Autodesk Inventor part; units mm, degrees
ref_plane "YZ Plane" through (0, 0, 0) normal (1, 0, 0) x (0, 1, 0)
ref_plane "XZ Plane" through (0, 0, 0) normal (0, 1, 0) x (-1, 0, 0)
ref_plane "XY Plane" through (0, 0, 0) normal (0, 0, 1) x (1, 0, 0)
sketch "Sketch1" plane through (0, 0, 0) normal (0, 0, 1) x (1, 0, 0)
  line L0 (-131, -26) -> (-49, -26) construction
  line L1 (-49, -26) -> (-49, -52.5) construction
  line L2 (-49, -52.5) -> (-131, -52.5) construction
  line L3 (-131, -52.5) -> (-131, -26) construction
  line L4 (-90, -26) -> (-90, 12) construction
  line L5 (-140, -12) -> (-40, -12) construction
  line L6 (-40, -12) -> (-40, -62) construction
  line L7 (-40, -62) -> (-140, -62) construction
  line L8 (-140, -62) -> (-140, -12) construction
  line L9 (-140, -18) -> (-40, -18) construction
  line L10 (-90, -12) -> (-90, 12) construction
  line L11 (0, 0) -> (-90, 0) construction
  line L12 (-30, -17.3205) -> (0, 34.641)
  line L13 (0, 34.641) -> (30, -17.3205)
  line L14 (30, -17.3205) -> (-30, -17.3205)
  line L15 (0, -17.3205) -> (0, 34.641) construction
  line L16 (-15, 8.6603) -> (30, -17.3205) construction
  line L17 (15, 8.6603) -> (-30, -17.3205) construction
  line L18 (80.3923, -115.2436) -> (30.3923, -28.641) construction
  line L19 (123.6936, -90.2436) -> (80.3923, -115.2436) construction
  line L20 (73.6936, -3.641) -> (123.6936, -90.2436) construction
  line L21 (30.3923, -28.641) -> (73.6936, -3.641) construction
  line L22 (67.5167, -64.9423) -> (34.6077, -83.9423) construction
  line L23 (59.6077, 127.2436) -> (9.6077, 40.641) construction
  line L24 (16.3064, 152.2436) -> (59.6077, 127.2436) construction
  line L25 (-33.6936, 65.641) -> (16.3064, 152.2436) construction
  line L26 (9.6077, 40.641) -> (-33.6936, 65.641) construction
  line L27 (22.4833, 90.9423) -> (55.3923, 71.9423) construction
  line L28 (3.9859, 170.9038) -> (-45, 86.0577)
  line L29 (-45, 86.0577) -> (-45, -11)
  line L30 (-45, -11) -> (-150, -11)
  line L31 (-150, -11) -> (-150, -82)
  line L32 (-52.0282, -82) -> (32.0263, -33.4711)
  line L33 (84.5263, -124.4038) -> (146.0141, -88.9038)
  line L34 (32.0263, -33.4711) -> (84.5263, -124.4038)
  line L35 (-150, -82) -> (-52.0282, -82)
  line L36 (97.0282, -4.0577) -> (12.9737, 44.4711)
  line L37 (65.4737, 135.4038) -> (3.9859, 170.9038)
  line L38 (12.9737, 44.4711) -> (65.4737, 135.4038)
  line L39 (146.0141, -88.9038) -> (97.0282, -4.0577)
  point P0 (-90, -18)
  point P1 (55.3923, -71.9423)
  point P2 (85.5885, -112.2436)
  point P3 (35.5885, -25.641)
  point P4 (110.9663, -87.1993)
  point P5 (69.9663, -16.1852)
  point P6 (47.0167, -29.4352)
  point P7 (88.0167, -100.4493)
  point P8 (34.6077, 83.9423)
  point P9 (54.4115, 130.2436)
  point P10 (4.4115, 43.641)
  point P11 (20.0337, 139.6993)
  point P12 (-20.9663, 68.6852)
  point P13 (1.9833, 55.4352)
  point P14 (42.9833, 126.4493)
  point P15 (3.9859, 170.9038)
  point P16 (-150, -82)
  point P17 (146.0141, -88.9038)
  dimension "d0" = 26.5
  dimension "d1" = 82
  dimension "d2" = 9.5
  dimension "d3" = 100
  dimension "d4" = 50
  dimension "d5" = 6
  dimension "d6" = 30
  dimension "d7" = 90
  dimension "d8" = 60
  dimension "d11" = 360
  dimension "d13" = 20
  dimension "d14" = 1
  dimension "d15" = 10
  dimension "d16" = 20
  dimension "d17" = 10
  dimension "d18" = 5
  dimension "d21" = 360
extrude "Extrusion1" add sketch "Sketch1" along normal blind 6
hole "Hole1" at (-131, -26, 0) at (-49, -26, 0) at (-49, -52.5, 0) at (-131, -52.5, 0) at (110.9663, -87.1993, 0) at (69.9663, -16.1852, 0) at (47.0167, -29.4352, 0) at (88.0167, -100.4493, 0) at (20.0337, 139.6993, 0) at (-20.9663, 68.6852, 0) at (1.9833, 55.4352, 0) at (42.9833, 126.4493, 0) direction (0, 0, 1) diameter 6.6 end through all
chamfer "Chamfer1" distance 7.5 angle 45 3 edges at (32.0263, -33.4711, 3) (12.9737, 44.4711, 3) (-45, -11, 3)
fillet "Fillet1" radius 10 6 edges at (84.5263, -124.4038, 3) (146.0141, -88.9038, 3) (-52.0282, -82, 3) (35.7763, -39.9663, 3) (25.5311, -37.2211, 3) (30, -17.3205, 3)
pattern_circular "Circular Pattern1" count 3 over 360 about axis through (0, 0, -10) along (0, 0, 1) of "Fillet1"
sketch "Sketch2" plane through (0, 0, 6) normal (0, 0, 1) x (1, 0, 0)
  point P0 (0, 0)
sketch "Sketch3" plane through (0, 0, 0) normal (0, 0, -1) x (-1, 0, 0)
  line L0 (-94.7077, -2.718) -> (-23.0561, 38.6501)
  line L1 (-141.0141, -80.2436) -> (-98.3679, -6.3782)
  line L2 (-93.1865, -119.4038) -> (-137.3538, -93.9038)
  line L3 (-8.6603, 19.641) -> (-21.3397, -2.3205)
  line L4 (-37.8473, -43.5535) -> (-79.5263, -115.7436)
  line L5 (-18.7948, 54.5535) -> (-60.4737, 126.7436)
  line L6 (-123.6936, -90.2436) -> (-113.6936, -72.923)
  line L7 (-113.6936, -72.923) -> (-131.0141, -62.923)
  line L8 (-131.0141, -62.923) -> (-141.0141, -80.2436)
  line L9 (-141.0141, -80.2436) -> (-123.6936, -90.2436)
  line L10 (-123.6936, -90.2436) -> (-131.0141, -62.923) construction
  line L11 (-113.6936, -72.923) -> (-141.0141, -80.2436) construction
  point P0 (0, 0)
  point P1 (-117.3538, -59.2628)
  point P2 (-127.3538, -76.5833)
  point P3 (-33.9545, 20.8109)
  point P4 (-16.634, 30.8109)
  point P5 (-38.6603, -12.3205)
  dimension "d39" = 10
  dimension "d40" = 10
  dimension "d41" = 20
  dimension "d42" = 20
  dimension "d43" = 10
  dimension "d44" = 10
  dimension "d46" = 10
  dimension "d47" = 20
  dimension "d49" = 120
  dimension "d50" = 30
  dimension "d58" = 20
  dimension "d59" = 20
hole "Hole2" at (38.6603, -12.3205, 0) at (33.9545, 20.8109, 0) at (16.634, 30.8109, 0) at (127.3538, -76.5833, 0) at (117.3538, -59.2628, 0) direction (0, 0, 1) diameter 5.5 end through all
pattern_circular "Circular Pattern2" count 3 over 360 about axis through (0, 0, -10) along (0, 0, 1) of "Hole2"
properties part number "RT_FRM_MC_V3_MotorBase"
Model file for the job. Use its own axes, mm. A direction names the side the tool comes from. Give positions to 0.01 mm unless a question says otherwise; leave off trailing zeros. Loops run counter-clockwise (first coordinate to the right, second up) from the corner with the lowest first, then second, coordinate; pieces in that order, holes last. Notation, with made-up numbers: (-22.5, -24) - (36.5, -24) arc R29 cw to (36.5, 11) - close; hole circle Ø9 at (89.5, 62). An arc over 180 degrees is marked (long way). Use one line per item in the form item = value.
(1) Cut at C-C (x = -99.5). Give the cut face in (y, z), then the cut area to 3 significant figures.
Determined:
outline = (-82, 0) - (-11, 0) - (-11, 6) - (-82, 6) - close
area = 426 mm^2
(2) Pull direction X, two halves, no side cores. Call faces 5 (the face through (-127.78, -53.22, 3.04)), 6 (the face through (-147.15, -78.99, 3.04)), 7 (the face through (35, 153, 3)): pulls with the +X half, pulls with the -X half, needs draft (parallel to the pull), parting line crosses it, or undercut.
Determined:
face_5 = undercut
face_6 = pulls with the -X half
face_7 = pulls with the +X half
(3) Cut at B-B (z = 4.85). Count the separate pieces of the cut face and the enclosed holes in it, then the cut area to 3 significant figures.
Determined:
separate_pieces = 1
enclosed_holes = 28
area = 30,700 mm^2
(4) Drill centre lines: L1, parallel to Y at x = -130.5, z = 5.25; L2, parallel to X at y = 56, z = 3.7; L3, parallel to X at y = -52.5, z = 2.45. Where is each one in solid material? Low to high.
Determined:
L1 = -82 to -74.7, -69.3 to -55.76, -49.24 to -29.26, -22.74 to -11
L2 = -45 to -1.27, 5.23 to 19.63
L3 = -150 to -134.3, -127.7 to -52.3, -45.7 to -0.93, 43.01 to 125
(5) Drop flat-ended pins along their axis: P1, Ø1, axis at y = 109.5, z = 2.5, coming from the -X side; P2, Ø3, axis at x = -118, z = 2.5, coming from the -Y side; P3, Ø1.8, axis at x = -4.5, z = 2, coming from the +Y side. Give the stop position or say it passes through.
Determined:
P1 = -31.75
P2 = -82
P3 = 157.76
(6) 3-axis set-ups, long thin cutter, end or side, ignore diameter. For faces 1 (the face through (58.395, -79.143, 2.958)), 2 (the face through (-22.039, 125.828, 2.958)), 3 (the face through (59.38, 17.68, 2.96)), 4 (the face through (-15.089, 8.507, 2.958)): which of +Z, -Z, +X, -X, +Y, -Y reach the whole face in a straight line?
Determined:
face_1 = +Z, -Z, -Y
face_2 = +Z, -Z, -X, +Y
face_3 = +Z, -Z, +X
face_4 = +Z, -Z
(7) Cut at A-A (y = -52.5). Give the cut face in (x, z), then the cut area to 3 significant figures.
Determined:
outline = (-150, 0) - (-134.3, 0) - (-134.3, 6) - (-150, 6) - close; (-127.7, 0) - (-52.3, 0) - (-52.3, 6) - (-127.7, 6) - close; (-45.7, 0) - (-0.93, 0) - (-0.93, 6) - (-45.7, 6) - close; (43.01, 0) - (125, 0) - (125, 6) - (43.01, 6) - close
area = 1,310 mm^2
